from build123d import *

# Parameters (mm, degrees)
SKETCH2_R           = 3.5685
SKETCH2_R_2         = 2.500000207
SKETCH2_R_3         = 2.500000038
SKETCH2_R_4         = 2.492850486
SKETCH2_R_5         = 1.499992866
SKETCH2_R_6         = 2.500000001
SKETCH2_R_7         = 2.492850485
BOSS_EXTRUDE1_DEPTH = 2.54


with BuildPart() as part:
    # Sketch2 → Boss-Extrude1 (new body)
    with BuildSketch(Plane.XY):
        with BuildLine():
            Line((-92.273812965, -51.714849286), (-14.273812965, -51.714848152))
            ThreePointArc((-14.273812965, -51.714848152), (-10.738279038, -53.179314194), (-9.273812892, -56.714848078))
            Line((-9.273812892, -56.714848078), (-9.273811154, -173.715325349))
            ThreePointArc((-9.273811154, -173.715325349), (-10.738277196, -177.250859277), (-14.273811081, -178.715325423))
            Line((-14.273811081, -178.715325423), (-92.273811081, -178.715326558))
            ThreePointArc((-92.273811081, -178.715326558), (-95.809345008, -177.250860516), (-97.273811154, -173.715326632))
            Line((-97.273811154, -173.715326632), (-97.273812892, -56.714849361))
            ThreePointArc((-97.273812892, -56.714849361), (-95.80934685, -53.179315433), (-92.273812965, -51.714849286))
        make_face()
        with Locations((-83.593812773, -64.894849171)):
            Circle(SKETCH2_R, mode=Mode.SUBTRACT)
        with Locations((-73.598714259, -64.889947536)):
            Circle(SKETCH2_R_2, mode=Mode.SUBTRACT)
        with Locations((-53.273812773, -64.894848719)):
            Circle(SKETCH2_R, mode=Mode.SUBTRACT)
        with Locations((-32.948911283, -64.88994693)):
            Circle(SKETCH2_R_2, mode=Mode.SUBTRACT)
        with Locations((-22.953812773, -64.894848267)):
            Circle(SKETCH2_R, mode=Mode.SUBTRACT)
        with Locations((-83.593812773, -74.894849171)):
            Circle(SKETCH2_R, mode=Mode.SUBTRACT)
        with Locations((-73.598714077, -74.894848647)):
            Circle(SKETCH2_R_3, mode=Mode.SUBTRACT)
        with Locations((-53.273812773, -74.894848719)):
            Circle(SKETCH2_R, mode=Mode.SUBTRACT)
        with Locations((-32.948911213, -74.89484821)):
            Circle(SKETCH2_R_3, mode=Mode.SUBTRACT)
        with Locations((-22.953812773, -74.894848267)):
            Circle(SKETCH2_R, mode=Mode.SUBTRACT)
        with Locations((-22.953812773, -84.894848267)):
            Circle(SKETCH2_R, mode=Mode.SUBTRACT)
        with Locations((-32.948911064, -84.89484821)):
            Circle(SKETCH2_R_3, mode=Mode.SUBTRACT)
        with Locations((-43.273812429, -84.894848364)):
            Circle(SKETCH2_R_3, mode=Mode.SUBTRACT)
        with Locations((-53.273812773, -84.894848719)):
            Circle(SKETCH2_R, mode=Mode.SUBTRACT)
        with Locations((-83.593812773, -84.894849171)):
            Circle(SKETCH2_R, mode=Mode.SUBTRACT)
        with Locations((-73.611151054, -84.902029225)):
            Circle(SKETCH2_R_4, mode=Mode.SUBTRACT)
        with Locations((-63.273812446, -84.894849)):
            Circle(SKETCH2_R_3, mode=Mode.SUBTRACT)
        with Locations((-83.593812773, -94.894849171)):
            Circle(SKETCH2_R, mode=Mode.SUBTRACT)
        with Locations((-73.598713779, -94.894848647)):
            Circle(SKETCH2_R_3, mode=Mode.SUBTRACT)
        with Locations((-63.433812595, -94.89485049)):
            Circle(SKETCH2_R_3, mode=Mode.SUBTRACT)
        with Locations((-53.273812773, -94.894848719)):
            Circle(SKETCH2_R, mode=Mode.SUBTRACT)
        with Locations((-68.09381174, -100.389947487)):
            Circle(SKETCH2_R_2, mode=Mode.SUBTRACT)
        with Locations((-91.293819406, -91.965099732)):
            Circle(SKETCH2_R_5, mode=Mode.SUBTRACT)
        with Locations((-91.293819406, -98.465072086)):
            Circle(SKETCH2_R_5, mode=Mode.SUBTRACT)
        with Locations((-91.293819108, -111.965103757)):
            Circle(SKETCH2_R_5, mode=Mode.SUBTRACT)
        with Locations((-83.593812304, -105.214849125)):
            Circle(SKETCH2_R_3, mode=Mode.SUBTRACT)
        with Locations((-73.593812423, -105.050424838)):
            Circle(SKETCH2_R_3, mode=Mode.SUBTRACT)
        with Locations((-73.598713476, -115.214848518)):
            Circle(SKETCH2_R_3, mode=Mode.SUBTRACT)
        with Locations((-63.273811994, -115.214848871)):
            Circle(SKETCH2_R_3, mode=Mode.SUBTRACT)
        with Locations((-53.273812023, -115.214848719)):
            Circle(SKETCH2_R_6, mode=Mode.SUBTRACT)
        with Locations((-53.273812447, -105.214848674)):
            Circle(SKETCH2_R_3, mode=Mode.SUBTRACT)
        with Locations(Location((-15.253806438, -111.965103757, 0), (0, 0, 180))):
            Circle(SKETCH2_R_5, mode=Mode.SUBTRACT)
        with Locations(Location((-15.25380614, -91.965099732, 0), (0, 0, 180))):
            Circle(SKETCH2_R_5, mode=Mode.SUBTRACT)
        with Locations(Location((-15.25380614, -98.465072086, 0), (0, 0, 180))):
            Circle(SKETCH2_R_5, mode=Mode.SUBTRACT)
        with Locations(Location((-22.953812773, -94.894849171, 0), (0, 0, 180))):
            Circle(SKETCH2_R, mode=Mode.SUBTRACT)
        with Locations(Location((-22.953813242, -105.214849125, 0), (0, 0, 180))):
            Circle(SKETCH2_R_3, mode=Mode.SUBTRACT)
        with Locations(Location((-32.948911767, -94.894848647, 0), (0, 0, 180))):
            Circle(SKETCH2_R_3, mode=Mode.SUBTRACT)
        with Locations(Location((-32.953813123, -105.050424838, 0), (0, 0, 180))):
            Circle(SKETCH2_R_3, mode=Mode.SUBTRACT)
        with Locations(Location((-38.453813806, -100.389947487, 0), (0, 0, 180))):
            Circle(SKETCH2_R_2, mode=Mode.SUBTRACT)
        with Locations(Location((-43.113812951, -94.89485049, 0), (0, 0, 180))):
            Circle(SKETCH2_R_3, mode=Mode.SUBTRACT)
        with Locations((-43.273811978, -115.214848235)):
            Circle(SKETCH2_R_3, mode=Mode.SUBTRACT)
        with Locations((-32.948910612, -115.214848081)):
            Circle(SKETCH2_R_3, mode=Mode.SUBTRACT)
        with Locations((-15.25380614, -138.464597304)):
            Circle(SKETCH2_R_5, mode=Mode.SUBTRACT)
        with Locations((-15.25380614, -131.96462495)):
            Circle(SKETCH2_R_5, mode=Mode.SUBTRACT)
        with Locations((-15.253806438, -118.464593279)):
            Circle(SKETCH2_R_5, mode=Mode.SUBTRACT)
        with Locations((-22.953813242, -125.214847911)):
            Circle(SKETCH2_R_3, mode=Mode.SUBTRACT)
        with Locations((-22.953812773, -135.534847865)):
            Circle(SKETCH2_R, mode=Mode.SUBTRACT)
        with Locations(Location((-22.953812773, -145.534848769, 0), (0, 0, 180))):
            Circle(SKETCH2_R, mode=Mode.SUBTRACT)
        with Locations(Location((-22.953812773, -155.534848769, 0), (0, 0, 180))):
            Circle(SKETCH2_R, mode=Mode.SUBTRACT)
        with Locations(Location((-22.953812773, -165.534848769, 0), (0, 0, 180))):
            Circle(SKETCH2_R, mode=Mode.SUBTRACT)
        with Locations(Location((-32.948911283, -165.539750106, 0), (0, 0, 180))):
            Circle(SKETCH2_R_2, mode=Mode.SUBTRACT)
        with Locations(Location((-32.948911213, -155.534848826, 0), (0, 0, 180))):
            Circle(SKETCH2_R_3, mode=Mode.SUBTRACT)
        with Locations(Location((-32.948911064, -145.534848826, 0), (0, 0, 180))):
            Circle(SKETCH2_R_3, mode=Mode.SUBTRACT)
        with Locations((-32.948911767, -135.534848389)):
            Circle(SKETCH2_R_3, mode=Mode.SUBTRACT)
        with Locations((-38.453813806, -130.039749549)):
            Circle(SKETCH2_R_2, mode=Mode.SUBTRACT)
        with Locations((-32.953813123, -125.379272198)):
            Circle(SKETCH2_R_3, mode=Mode.SUBTRACT)
        with Locations((-43.113812951, -135.534846546)):
            Circle(SKETCH2_R_3, mode=Mode.SUBTRACT)
        with Locations(Location((-43.273812429, -145.534848672, 0), (0, 0, 180))):
            Circle(SKETCH2_R_3, mode=Mode.SUBTRACT)
        with Locations(Location((-53.273812773, -165.534848317, 0), (0, 0, 180))):
            Circle(SKETCH2_R, mode=Mode.SUBTRACT)
        with Locations(Location((-53.273812773, -155.534848317, 0), (0, 0, 180))):
            Circle(SKETCH2_R, mode=Mode.SUBTRACT)
        with Locations(Location((-53.273812773, -145.534848317, 0), (0, 0, 180))):
            Circle(SKETCH2_R, mode=Mode.SUBTRACT)
        with Locations(Location((-53.273812773, -135.534848317, 0), (0, 0, 180))):
            Circle(SKETCH2_R, mode=Mode.SUBTRACT)
        with Locations(Location((-53.273812447, -125.214848362, 0), (0, 0, 180))):
            Circle(SKETCH2_R_3, mode=Mode.SUBTRACT)
        with Locations(Location((-63.273812446, -145.534848036, 0), (0, 0, 180))):
            Circle(SKETCH2_R_3, mode=Mode.SUBTRACT)
        with Locations(Location((-63.433812595, -135.534846546, 0), (0, 0, 180))):
            Circle(SKETCH2_R_3, mode=Mode.SUBTRACT)
        with Locations(Location((-68.09381174, -130.039749549, 0), (0, 0, 180))):
            Circle(SKETCH2_R_2, mode=Mode.SUBTRACT)
        with Locations(Location((-73.593812423, -125.379272198, 0), (0, 0, 180))):
            Circle(SKETCH2_R_3, mode=Mode.SUBTRACT)
        with Locations(Location((-73.598713779, -135.534848389, 0), (0, 0, 180))):
            Circle(SKETCH2_R_3, mode=Mode.SUBTRACT)
        with Locations(Location((-73.611151054, -145.527667811, 0), (0, 0, 180))):
            Circle(SKETCH2_R_7, mode=Mode.SUBTRACT)
        with Locations(Location((-73.598714077, -155.534848389, 0), (0, 0, 180))):
            Circle(SKETCH2_R_3, mode=Mode.SUBTRACT)
        with Locations(Location((-73.598714259, -165.5397495, 0), (0, 0, 180))):
            Circle(SKETCH2_R_2, mode=Mode.SUBTRACT)
        with Locations(Location((-91.293819406, -138.464597304, 0), (0, 0, 180))):
            Circle(SKETCH2_R_5, mode=Mode.SUBTRACT)
        with Locations(Location((-91.293819406, -131.96462495, 0), (0, 0, 180))):
            Circle(SKETCH2_R_5, mode=Mode.SUBTRACT)
        with Locations(Location((-91.293819108, -118.464593279, 0), (0, 0, 180))):
            Circle(SKETCH2_R_5, mode=Mode.SUBTRACT)
        with Locations(Location((-83.593812304, -125.214847911, 0), (0, 0, 180))):
            Circle(SKETCH2_R_3, mode=Mode.SUBTRACT)
        with Locations(Location((-83.593812773, -135.534847865, 0), (0, 0, 180))):
            Circle(SKETCH2_R, mode=Mode.SUBTRACT)
        with Locations(Location((-83.593812773, -145.534847865, 0), (0, 0, 180))):
            Circle(SKETCH2_R, mode=Mode.SUBTRACT)
        with Locations(Location((-83.593812773, -155.534847865, 0), (0, 0, 180))):
            Circle(SKETCH2_R, mode=Mode.SUBTRACT)
        with Locations(Location((-83.593812773, -165.534847865, 0), (0, 0, 180))):
            Circle(SKETCH2_R, mode=Mode.SUBTRACT)
    extrude(amount=BOSS_EXTRUDE1_DEPTH)


solid = part.part
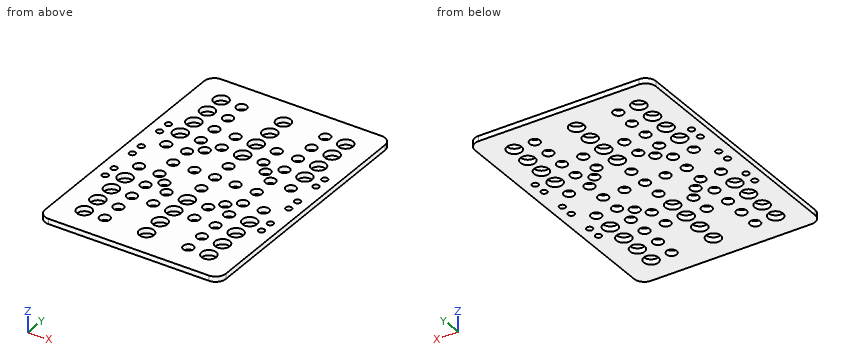
Work out the finished part from the listing and answer in its coordinate system (mm). Coordinates: 2 decimals unless noted, no trailing zeros. Write each loop counter-clockwise with the first axis right and the second up, starting at its lowest first coordinate (ties: lowest second). Pieces come first, ordered by that corner, then holes. Notation, with made-up numbers: M 3,70 L 38,70 A7 cw 38,83 Z; hole C -14.5,10.25 d5. An arc over 180 degrees is marked long. Use one line per item in the form item = value. Start each with the question number.
1. The part is cut by section A-A (x = -37.5). Give the vertices of the cut face in (y, z), plus the area to 3 significant figures.
2. This flat-tipped pin is pushed along its axis until it touches: P1, Ø11.5, axis at x = -22.95, y = -155.53, coming from the -Z side. Where does it stop, or does it pass through?
3. Straight lines are drawn through the part: probe 1 along X at (y, z) = (-125, 2.05); probe 2 along X at (y, z) = (-129.5, 0.4); probe 3 along X at (y, z) = (-166.5, 2.45). For each, find the intervals that lie inside material, in ascending order. Write a range as from..to.
4. The part is cut by section B-B (z = 1.4). Give the number of separate pieces and of enclosed holes in the cut face, plus the area to 3 significant figures.
Evaluation:
q1.outline = M -178.72,0 L -132.35,0 L -132.35,2.54 L -178.72,2.54 Z; M -127.73,0 L -102.7,0 L -102.7,2.54 L -127.73,2.54 Z; M -98.08,0 L -51.71,0 L -51.71,2.54 L -98.08,2.54 Z
q1.area = 299 mm^2
q2.P1 = 0
q3.probe_1 = -97.27..-86.08, -81.1..-76.06, -71.12..-55.76, -50.78..-35.42, -30.48..-25.44, -20.46..-9.27
q3.probe_2 = -97.27..-70.53, -65.65..-40.89, -36.01..-9.27
q3.probe_3 = -97.27..-87.03, -80.16..-75.91, -71.29..-56.71, -49.84..-35.26, -30.64..-26.39, -19.52..-9.27
q4.separate_pieces = 1
q4.enclosed_holes = 79
q4.area = 9,270 mm^2
